```python
from build123d import *

# Parameters (mm, degrees)
SKETCH1_R           = 23.5
SKETCH1_R_2         = 1.5
SKETCH1_R_3         = 1
BOSS_EXTRUDE1_DEPTH = 4
SKETCH2_R           = 2.7
CUT_EXTRUDE1_DEPTH  = 1.5
SKETCH3_R           = 2.5
CUT_EXTRUDE2_DEPTH  = 1
SKETCH4_R           = 3.7
SKETCH4_R_2         = 2.7
EXTRUDE_THIN1_DEPTH = 1


with BuildPart() as part:
    # Sketch1 → Boss-Extrude1 (new body)
    with BuildSketch(Plane(origin=(0, 0, 0), x_dir=(1, 0, 0), z_dir=(0, 1, 0))):
        Circle(SKETCH1_R)
        Circle(SKETCH1_R_2, mode=Mode.SUBTRACT)
        with Locations((0, 20)):
            Circle(SKETCH1_R_3, mode=Mode.SUBTRACT)
        with Locations((6.180339887, 19.021130326)):
            Circle(SKETCH1_R_3, mode=Mode.SUBTRACT)
        with Locations((11.755705046, 16.180339887)):
            Circle(SKETCH1_R_3, mode=Mode.SUBTRACT)
        with Locations((16.180339887, 11.755705046)):
            Circle(SKETCH1_R_3, mode=Mode.SUBTRACT)
        with Locations((19.021130326, 6.180339887)):
            Circle(SKETCH1_R_3, mode=Mode.SUBTRACT)
        with Locations((20, 0)):
            Circle(SKETCH1_R_3, mode=Mode.SUBTRACT)
        with Locations((19.021130326, -6.180339887)):
            Circle(SKETCH1_R_3, mode=Mode.SUBTRACT)
        with Locations((16.180339887, -11.755705046)):
            Circle(SKETCH1_R_3, mode=Mode.SUBTRACT)
        with Locations((11.755705046, -16.180339887)):
            Circle(SKETCH1_R_3, mode=Mode.SUBTRACT)
        with Locations((6.180339887, -19.021130326)):
            Circle(SKETCH1_R_3, mode=Mode.SUBTRACT)
        with Locations((0, -20)):
            Circle(SKETCH1_R_3, mode=Mode.SUBTRACT)
        with Locations((-6.180339887, -19.021130326)):
            Circle(SKETCH1_R_3, mode=Mode.SUBTRACT)
        with Locations((-11.755705046, -16.180339887)):
            Circle(SKETCH1_R_3, mode=Mode.SUBTRACT)
        with Locations((-16.180339887, -11.755705046)):
            Circle(SKETCH1_R_3, mode=Mode.SUBTRACT)
        with Locations((-19.021130326, -6.180339887)):
            Circle(SKETCH1_R_3, mode=Mode.SUBTRACT)
        with Locations((-20, 0)):
            Circle(SKETCH1_R_3, mode=Mode.SUBTRACT)
        with Locations((-19.021130326, 6.180339887)):
            Circle(SKETCH1_R_3, mode=Mode.SUBTRACT)
        with Locations((-16.180339887, 11.755705046)):
            Circle(SKETCH1_R_3, mode=Mode.SUBTRACT)
        with Locations((-11.755705046, 16.180339887)):
            Circle(SKETCH1_R_3, mode=Mode.SUBTRACT)
        with Locations((-6.180339887, 19.021130326)):
            Circle(SKETCH1_R_3, mode=Mode.SUBTRACT)
        with Locations((0, 12.191930978)):
            Circle(SKETCH1_R_2, mode=Mode.SUBTRACT)
        with Locations((12.191930978, 0)):
            Circle(SKETCH1_R_2, mode=Mode.SUBTRACT)
        with Locations((0, -12.191930978)):
            Circle(SKETCH1_R_2, mode=Mode.SUBTRACT)
        with Locations((-12.191930978, 0)):
            Circle(SKETCH1_R_2, mode=Mode.SUBTRACT)
        with Locations((-8.4255338, 8.4255338)):
            Circle(SKETCH1_R_3, mode=Mode.SUBTRACT)
        with Locations((8.4255338, 8.4255338)):
            Circle(SKETCH1_R_3, mode=Mode.SUBTRACT)
        with Locations((8.4255338, -8.4255338)):
            Circle(SKETCH1_R_3, mode=Mode.SUBTRACT)
        with Locations((-8.4255338, -8.4255338)):
            Circle(SKETCH1_R_3, mode=Mode.SUBTRACT)
    extrude(amount=BOSS_EXTRUDE1_DEPTH)

    # Sketch2 → Cut-Extrude1 (cut)
    with BuildSketch(Plane.XZ):
        Circle(SKETCH2_R)
    extrude(amount=-CUT_EXTRUDE1_DEPTH, mode=Mode.SUBTRACT)

    # Sketch3 → Cut-Extrude2 (cut)
    with BuildSketch(Plane(origin=(0, 4, 0), x_dir=(1, 0, 0), z_dir=(0, 1, 0))):
        Circle(SKETCH3_R)
    extrude(amount=-CUT_EXTRUDE2_DEPTH, mode=Mode.SUBTRACT)

    # Sketch4 → Extrude-Thin1 (add)
    with BuildSketch(Plane.XZ):
        Circle(SKETCH4_R)
        Circle(SKETCH4_R_2, mode=Mode.SUBTRACT)
    extrude(amount=EXTRUDE_THIN1_DEPTH)


solid = part.part
```
Design review of the part built by this model. Coordinates are the model's own, in mm. A direction names the side the tool comes from. Coordinates: 2 decimals unless noted, no trailing zeros. Order: outer loops, then holes, each group sorted by start corner. A loop starts at its lowest first (then second) coordinate and runs counter-clockwise, first axis right, second up. Notation, with made-up numbers: (14, 22.25) - (63, 22.25) arc R36 ccw to (63, 59.25) - close; hole circle Ø6 at (-10, 7.5). An arc over 180 degrees is marked (long way). One line per question, with ' | ' between items.
Q1. Consider section B-B, the plane y = 2.2. Give the number of separate pieces and of enclosed holes in the cut face, then the cut area to 3 significant figures.
Answer key:
separate pieces: 1 | enclosed holes: 29 | area: 1,620 mm2
Q2. Clearance check with flat-ended pins moving along their axes: pin 1 Ø2 at (x, y) = (-1.5, 3) entering from +Z; pin 2 Ø2 at (y, z) = (2, -6) entering from -X; pin 3 Ø1.5 at (x, y) = (-8.5, -0.5) entering from -Z; pin 4 Ø2.5 at (x, z) = (-6.18, 19.02) entering from +Y. State where each tip first meets the part, or that it passes through.
Answer key:
pin 1: stops at z = 23.49 | pin 2: stops at x = -22.96 | pin 3: stops at z = -22.12 | pin 4: stops at y = 4
Q3. For faces 4 (the cylindrical face through (9.38, 1.97, -8.73)), 5 (the flat face through (1.2, 1.5, -1.2)), 6 (the flat face through (0, 3, 2)), list the 3-axis set-ups (+Z, -Z, +X, -X, +Y, -Y) from which the entire face can be reached by the end or side of a thin tool; tool diameter is ignored.
Answer key:
face 4: +Y, -Y | face 5: -Y | face 6: +Y
Q4. To check wall thickness, follow line 1 along Z through (x, y) = (-6, 2.8); line 2 along Z through (x, y) = (-12, 2.15). State the ranges of each line that lie inside material, in increasing order.
Answer key:
line 1: z = -22.72 to -20, -18.04 to 18.04, 20 to 22.72 | line 2: z = -20.21 to -17.15, -15.21 to -1.49, 1.49 to 15.21, 17.15 to 20.21
Q5. Consider section C-C, the plane x = -6. Give the boundary of the cut face in (y, z).
Answer key:
outline: (0, -22.72) - (4, -22.72) - (4, -20) - (0, -20) - close; (0, -18.04) - (4, -18.04) - (4, 18.04) - (0, 18.04) - close; (0, 20) - (4, 20) - (4, 22.72) - (0, 22.72) - close
Q6. The part is to be moulded in two halves that separate along X. For faces 1 (the cylindrical face through (15.387, 1.972, -11.147)), 2 (the flat face through (0, 0, 5)), 3 (the cylindrical face through (-0.802, -0.493, -3.612)), say which applies: +X half, -X half, draft (parallel to the pull), parting line (faces both ways), or undercut.
Answer key:
face 1: undercut | face 2: draft | face 3: parting line
Q7. Consider section A-A, the plane x = 12. Give the boundary of the cut face in (y, z).
Answer key:
outline: (0, -20.21) - (4, -20.21) - (4, -17.15) - (0, -17.15) - close; (0, -15.21) - (4, -15.21) - (4, -1.49) - (0, -1.49) - close; (0, 1.49) - (4, 1.49) - (4, 15.21) - (0, 15.21) - close; (0, 17.15) - (4, 17.15) - (4, 20.21) - (0, 20.21) - close
